```python
from build123d import *

# Parameters (mm, degrees)
F1_DEPTH = 35.56
F3_DEPTH = 7.001
F4_R     = 15.24
F5_R     = 5.08
F6_R     = 2.25
F7_DEPTH = 5.001
F8_SIZE2 = 8.7988181024
F8_SIZE  = 15.24


with BuildPart() as f1:
    # F0 (on Top) → F1 (new body, symmetric)
    with BuildSketch(Plane.XY):
        Polygon((0, 0), (-78.74, 0), (-78.74, 4), (-82.74, 4), (-82.74, -7), (5, -7), (5, 38.72), (0, 38.72), align=None)
    extrude(amount=F1_DEPTH, both=True)

    # F2 (on face) → F3 (cut, through all)
    with BuildSketch(Plane(origin=(0, 0, 0), x_dir=(-1, 0, 0), z_dir=(0, 1, 0))):
        Polygon((77.34, 15.3979316793), (50.67, 30.7958633586), (24, 15.3979316793), (24, -15.3979316793), (50.67, -30.7958633586), (77.34, -15.3979316793), align=None)
    extrude(amount=-F3_DEPTH, mode=Mode.SUBTRACT)

    # F4
    f4_edges = [f1.edges().sort_by_distance(p)[0] for p in [
        (0, 0, 0),
    ]]
    fillet(f4_edges, radius=F4_R)

    # F5
    f5_edges = [f1.edges().sort_by_distance(p)[0] for p in [
        (5, -7, 0),
    ]]
    fillet(f5_edges, radius=F5_R)

    # F6 (on face) → F7 (cut, through all)
    with BuildSketch(Plane(origin=(0, 0, 0), x_dir=(0, -1, 0), z_dir=(-1, 0, 0))):
        with Locations((-23.48, 25.11)):
            Circle(F6_R)
        with Locations((-23.48, -22.86)):
            Circle(F6_R)
    extrude(amount=-F7_DEPTH, mode=Mode.SUBTRACT)

    # F8
    f8_edges = [f1.edges().sort_by_distance(p)[0] for p in [
        (2.5, 38.72, 35.56),
        (2.5, 38.72, -35.56),
    ]]
    f8_side = f1.faces().sort_by_distance((2.5, 38.72, 0))[0]
    chamfer(f8_edges, length=F8_SIZE, length2=F8_SIZE2, reference=f8_side)


solid = f1.part
```
Geometry: final body of the model. Coordinates: model frame, mm. A direction names the side the tool comes from. Coordinates: 2 decimals unless noted, no trailing zeros. Loops run counter-clockwise (first coordinate to the right, second up) from the corner with the lowest first, then second, coordinate; pieces in that order, holes last. Notation, with made-up numbers: M 40.5,-35.75 L 87.5,-35.75 A15 cw 87.5,-24.75 Z; hole C 85.25,-19 d5. An arc over 180 degrees is marked long. Put each result on its own line as item: value.
(1) Cut plane C-C on x = -30.5. Return the cut outline in (y, z).
Answer sheet:
outline: M -7,-35.56 L 0,-35.56 L 0,-19.15 L -7,-19.15 Z; M -7,19.15 L 0,19.15 L 0,35.56 L -7,35.56 Z
(2) First-contact query: pin 1 (1 mm diameter, centred on x = -32, z = -20.5, fed in from +Y); pin 2 (2 mm diameter, centred on y = -4, z = -1.5, fed in from +X); pin 3 (3 mm diameter, centred on x = -81, z = -7.5, fed in from +Y). Flat tips, straight axial feed; report the tip coordinate or a pass-through.
Answer sheet:
pin 1: stops at y = 0
pin 2: stops at x = 4.88
pin 3: stops at y = 4
(3) Access query for faces 5 (the face through (-81, 4, 0)), 6 (the face through (-37.522, -3.451, 23.205)), 7 (the face through (3, 38.72, 0)), 8 (the face through (-78.74, 2, 0)). Directions: +Z, -Z, +X, -X, +Y, -Y. A direction counts if a zero-diameter tool reaches every point of the face in a straight line with its end or side. Return the directions, or none.
Answer sheet:
face 5: +Z, -Z, -X, +Y
face 6: +Y, -Y
face 7: +Z, -Z, +X, -X, +Y
face 8: +Z, -Z, +Y
(4) Cut plane A-A on y = 23.48. Return the cut outline in (x, z).
Answer sheet:
outline: M 0,-35.56 L 5,-35.56 L 5,-25.11 L 0,-25.11 Z; M 0,-20.61 L 5,-20.61 L 5,22.86 L 0,22.86 Z; M 0,27.36 L 5,27.36 L 5,35.56 L 0,35.56 Z
(5) Draft query along X for faces 1 (the face through (5, 18, 0)), 2 (the face through (-4.58, 4.35, -0.5)), 3 (the face through (2.535, 34.259, -28.047)), 4 (the face through (-64.19, -3.45, 22.99)). Return one class per face: pulls with the +X half, pulls with the -X half, needs draft (parallel to the pull), parting line crosses it, or undercut.
Answer sheet:
face 1: pulls with the +X half
face 2: undercut
face 3: needs draft
face 4: undercut
(6) Material intervals for probe 1 along Z at (x, y) = (3.5, 23.48); probe 2 along Z at (x, y) = (3, 23); probe 3 along X at (y, z) = (31.5, -30), sorted ascending.
Answer sheet:
probe 1: z = -35.56 to -25.11, -20.61 to 22.86, 27.36 to 35.56
probe 2: z = -35.56 to -25.06, -20.66 to 22.91, 27.31 to 35.56
probe 3: x = 0 to 5
(7) Cut plane B-B on z = 29. Return the cut outline in (x, y), then the cut area to 3 significant figures.
Answer sheet:
outline: M -82.74,-7 L -53.78,-7 L -53.78,0 L -78.74,0 L -78.74,4 L -82.74,4 Z; M -47.56,-7 L -0.08,-7 A5.08 ccw 5,-1.92 L 5,33.71 L 0,33.71 L 0,15.24 A15.24 cw -15.24,0 L -47.56,0 Z
area: 799 mm^2
(8) Cut plane D-D on z = -22.86. Return the cut outline in (x, y).
Answer sheet:
outline: M -82.74,-7 L -64.42,-7 L -64.42,0 L -78.74,0 L -78.74,4 L -82.74,4 Z; M -36.92,-7 L -0.08,-7 A5.08 ccw 5,-1.92 L 5,21.23 L 0,21.23 L 0,15.24 A15.24 cw -15.24,0 L -36.92,0 Z; M 0,25.73 L 5,25.73 L 5,37.25 L 0,37.25 Z
